```python
from build123d import *

# Parameters (mm, degrees)
EXTRUDE_1_DEPTH = 3
FILLET_1_R      = 3
FILLET_2_R      = 2


with BuildPart() as part:
    # 草图1 → 凸台-拉伸1 (new body)
    with BuildSketch(Plane.XY):
        with BuildLine():
            Line((-30, -23), (-30, -28))
            Line((-30, -28), (-19, -28))
            Line((-19, -28), (-16, -31))
            Line((-16, -31), (16, -31))
            Line((16, -31), (19, -28))
            Line((19, -28), (30, -28))
            Line((30, -28), (30, -23))
            Line((30, -23), (30, -18))
            Line((30, -18), (30, -15.5))
            Line((30, -15.5), (33, -12.5))
            Line((33, -12.5), (33, 12.5))
            Line((33, 12.5), (30, 15.5))
            Line((30, 15.5), (30, 28))
            Line((30, 28), (-30, 28))
            Line((-30, 28), (-30, -6.9))
            ThreePointArc((-30, -6.9), (-29.25753788, -7.20753788), (-28.95, -7.95))
            ThreePointArc((-28.95, -7.95), (-29.25753788, -8.69246212), (-30, -9))
            Line((-30, -9), (-33, -9))
            Line((-33, -9), (-33, -19))
            Line((-33, -19), (-30, -19))
            ThreePointArc((-30, -19), (-29.25753788, -19.30753788), (-28.95, -20.05))
            ThreePointArc((-28.95, -20.05), (-29.25753788, -20.79246212), (-30, -21.1))
            Line((-30, -21.1), (-30, -23))
        make_face()
        with BuildLine():
            Line((25, -10.3), (25, -23))
            Line((25, -23), (13.2, -23))
            Line((13.2, -23), (13.2, -26))
            ThreePointArc((13.2, -26), (12.15, -27.05), (11.1, -26))
            Line((11.1, -26), (7.1, -26))
            ThreePointArc((7.1, -26), (6.05, -27.05), (5, -26))
            Line((5, -26), (5, -23))
            Line((5, -23), (-5, -23))
            Line((-5, -23), (-5, -26))
            ThreePointArc((-5, -26), (-6.05, -27.05), (-7.1, -26))
            Line((-7.1, -26), (-11.1, -26))
            ThreePointArc((-11.1, -26), (-12.15, -27.05), (-13.2, -26))
            Line((-13.2, -26), (-13.2, -23))
            Line((-13.2, -23), (-25, -23))
            Line((-25, -23), (-25, 23))
            Line((-25, 23), (25, 23))
            Line((25, 23), (25, 10.3))
            Line((25, 10.3), (28, 10.3))
            ThreePointArc((28, 10.3), (28.74246212, 9.99246212), (29.05, 9.25))
            ThreePointArc((29.05, 9.25), (28.74246212, 8.50753788), (28, 8.2))
            Line((28, 8.2), (28, 6.1))
            ThreePointArc((28, 6.1), (28.74246212, 5.79246212), (29.05, 5.05))
            ThreePointArc((29.05, 5.05), (28.74246212, 4.30753788), (28, 4))
            Line((28, 4), (25, 4))
            Line((25, 4), (25, -4))
            Line((25, -4), (28, -4))
            ThreePointArc((28, -4), (28.74246212, -4.30753788), (29.05, -5.05))
            ThreePointArc((29.05, -5.05), (28.74246212, -5.79246212), (28, -6.1))
            Line((28, -6.1), (28, -8.2))
            ThreePointArc((28, -8.2), (28.74246212, -8.50753788), (29.05, -9.25))
            ThreePointArc((29.05, -9.25), (28.74246212, -9.99246212), (28, -10.3))
            Line((28, -10.3), (25, -10.3))
        make_face(mode=Mode.SUBTRACT)
    extrude(amount=EXTRUDE_1_DEPTH)

    # 圆角1
    fillet_1_edges = [part.edges().sort_by_distance(p)[0] for p in [
        (-30, 28, 1.5),
        (30, 28, 1.5),
        (30, -28, 1.5),
        (-30, -28, 1.5),
    ]]
    fillet(fillet_1_edges, radius=FILLET_1_R)

    # 圆角2
    fillet_2_edges = [part.edges().sort_by_distance(p)[0] for p in [
        (25, 23, 1.5),
        (-25, 23, 1.5),
        (-25, -23, 1.5),
        (25, -23, 1.5),
    ]]
    fillet(fillet_2_edges, radius=FILLET_2_R)


solid = part.part
```
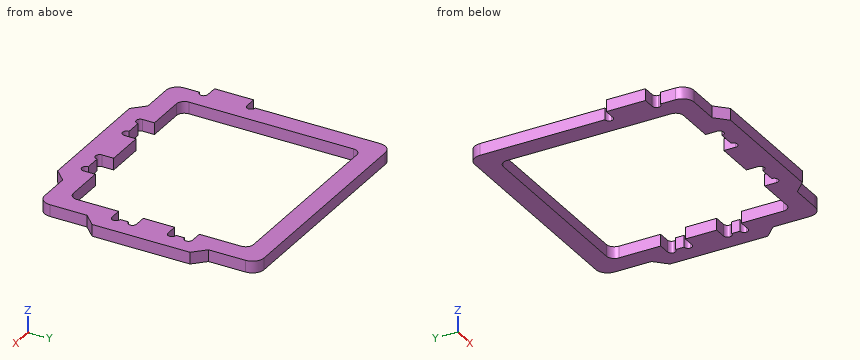
Design review of the part built by this model. Coordinates are the model's own, in mm. Round coordinates to 2 decimals unless told otherwise and drop trailing zeros. Write each loop counter-clockwise with the first axis right and the second up, starting at its lowest first coordinate (ties: lowest second). Pieces come first, ordered by that corner, then holes. Notation, with made-up numbers: (-4, 75.5) -> (21, 75.5) arc R25 ccw to (21, 92.5) -> close; hole circle Ø4 at (46, 78.25). An arc over 180 degrees is marked (long way). Answer in a Markdown table with one row per item.
Q1. Clearance check with flat-ended pins moving along their axes: pin 1 Ø0.9 at (y, z) = (16, 1) entering from -X; pin 2 Ø0.9 at (y, z) = (-21, 1.5) entering from +X; pin 3 Ø1.5 at (x, z) = (27, 1) entering from -Y. State where each tip first meets the part, or that it passes through.
The answers:
| item | result |
|---|---|
| pin 1 | x = -30 |
| pin 2 | x = 30 |
| pin 3 | y = -28 |
Q2. To check wall thickness, follow L1, parallel to X at y = 0.5, z = 1.1; L2, parallel to Y at x = 9.5, z = 0.6; L3, parallel to X at y = 17, z = 2.6. State the ranges of each line that lie inside material, in increasing order. Write a range as [from, to].
The answers:
| item | result |
|---|---|
| L1 | [-30, -25], [25, 33] |
| L2 | [-31, -26], [23, 28] |
| L3 | [-30, -25], [25, 30] |
Q3. Take a section at A-A, the plane y = -1. State the section outline as (x, z) points.
The answers:
| item | result |
|---|---|
| outline | (-30, 0) -> (-25, 0) -> (-25, 3) -> (-30, 3) -> close; (25, 0) -> (33, 0) -> (33, 3) -> (25, 3) -> close |
Q4. Take a section at B-B, the plane x = -12.15. State the section outline as (y, z) points, then the cut area to 4 significant figures.
The answers:
| item | result |
|---|---|
| outline | (-31, 0) -> (-27.05, 0) -> (-27.05, 3) -> (-31, 3) -> close; (23, 0) -> (28, 0) -> (28, 3) -> (23, 3) -> close |
| area | 26.85 mm² |
